For this review, use the dimensioned drawing (mm, ordinates from the lowest corner) and the shaded views. Give positions to 0.01 mm unless a question says otherwise; leave off trailing zeros. Order: outer loops, then holes, each group sorted by start corner. A loop starts at its lowest first (then second) coordinate and runs counter-clockwise, first axis right, second up.
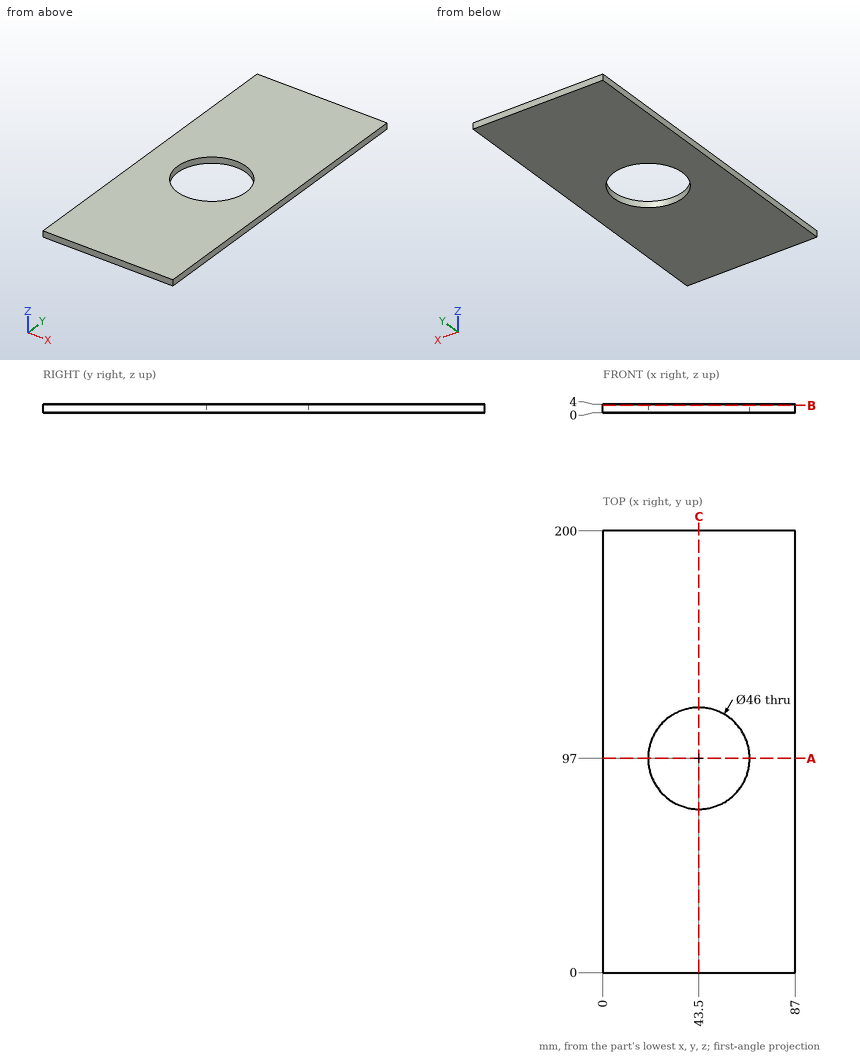
1. For line 1 along Y through (x, z) = (43.5, 1.7); line 2 along Y through (x, z) = (36, 3.85); line 3 along X through (y, z) = (91.5, 3.1), list the stretches that pass through material, from the lowest coordinate up.
Recorded:
line 1: y = 0 to 74, 120 to 200
line 2: y = 0 to 75.26, 118.74 to 200
line 3: x = 0 to 21.17, 65.83 to 87
2. Take a section at C-C (x = 43.5). State the section outline as (y, z) points, then the cut area to 3 significant figures.
Recorded:
outline: (0, 0) - (74, 0) - (74, 4) - (0, 4) - close; (120, 0) - (200, 0) - (200, 4) - (120, 4) - close
area: 616 mm2
3. Take a section at B-B (z = 3.35). State the section outline as (x, y) points.
Recorded:
outline: (0, 0) - (87, 0) - (87, 200) - (0, 200) - close; hole circle Ø46 at (43.5, 97)
4. Take a section at A-A (y = 97). State the section outline as (x, z) points, then the cut area to 3 significant figures.
Recorded:
outline: (0, 0) - (20.5, 0) - (20.5, 4) - (0, 4) - close; (66.5, 0) - (87, 0) - (87, 4) - (66.5, 4) - close
area: 164 mm2
